Part model, mm, in its own coordinate system. Face numbers are marked on the shaded views. A direction names the side the tool comes from. Coordinates: 2 decimals unless noted, no trailing zeros. Write each loop counter-clockwise with the first axis right and the second up, starting at its lowest first coordinate (ties: lowest second). Pieces come first, ordered by that corner, then holes. Notation, with made-up numbers: (88.5, -33) -> (108.5, -33) arc R17 ccw to (108.5, -27) -> close; hole circle Ø7 at (82.5, 83). An arc over 180 degrees is marked (long way). Write item = value, one per line. Start each with the question number.
Q1. Band-saw the part on A-A, the plane z = 1.75. List the corners of the cut face in (x, y), plus the area to 3 significant figures.
Q2. Band-saw the part on D-D, the plane z = -0.5. Give the number of separate pieces and of enclosed holes in the cut face, plus the area to 3 significant figures.
Q3. Pull direction X, two halves, no side cores. Call the marked faces 1, 2 and 3: released by +X, released by -X, zero draft, split by the parting line, or undercut.
Q4. Band-saw the part on C-C, the plane y = 2.55. List the corners of the cut face in (x, z).
Q5. Band-saw the part on B-B, the plane x = -1.25. List the corners of the cut face in (y, z), plus the area to 3 significant figures.
Q6. Probe line 1 (X direction, y = 0.65, z = 3); line 2 (Z direction, x = 4.25, y = 1.8). List the from-to ranges inside material, lowest first.
Q7. Tool access for the marked faces 4 and 5: list every direction of +Z, -Z, +X, -X, +Y, -Y with a clear straight run to the whole face (end or side of a thin tool).
Autodesk Inventor part; units mm, degrees
ref_plane "YZ Plane" through (0, 0, 0) normal (1, 0, 0) x (0, 1, 0)
ref_plane "XZ Plane" through (0, 0, 0) normal (0, 1, 0) x (-1, 0, 0)
ref_plane "XY Plane" through (0, 0, 0) normal (0, 0, 1) x (1, 0, 0)
sketch "Sketch1" plane through (0, 0, 0) normal (0, 1, 0) x (-1, 0, 0)
  line L0 (5, 5) -> (-5, 5)
  line L1 (-5, 5) -> (-5, -5)
  line L2 (-5, -5) -> (5, -5)
  line L3 (5, -5) -> (5, 5)
  line L4 (6, 6) -> (-6, 6)
  line L5 (-6, 6) -> (-6, -6)
  line L6 (-6, -6) -> (6, -6)
  line L7 (6, -6) -> (6, 6)
  point P0 (0, 0)
  dimension "d0" = 10
  dimension "d1" = 10
  dimension "d2" = 5
  dimension "d3" = 5
  dimension "d4" = 12
  dimension "d5" = 12
  dimension "d6" = 1
  dimension "d7" = 1
extrude "Extrusion1" add sketch "Sketch1" along normal blind 2
sketch "Sketch2" plane through (6, 0, 6) normal (1, 0, 0) x (0, 0, -1)
  line L0 (0, 0) -> (0, 2)
  line L1 (12, 0) -> (12, 2)
  line L2 (0, 2) -> (12, 2)
  line L3 (12, 2) -> (12, 1)
  line L4 (12, 1) -> (0, 1)
  line L5 (0, 1) -> (0, 2)
  point P0 (6, 0)
extrude "Extrusion2" add sketch "Sketch2" against normal blind 11.5
sketch "Sketch3" plane through (0, 2, 0) normal (0, 1, 0) x (1, 0, 0)
  line L0 (-2, -2) -> (2, -2)
  line L1 (2, -2) -> (2, 2)
  line L2 (2, 2) -> (-2, 2)
  line L3 (-2, 2) -> (-2, -2)
  circle A0 centre (0, 0) radius 2.8284
  line L4 (0, -2.8284) -> (-2.8284, 0)
  line L5 (-2.8284, 0) -> (0, 2.8284)
  line L6 (2.8284, 0) -> (0, 2.8284)
  line L7 (2.8284, 0) -> (0, -2.8284)
  point P0 (0.8284, -2)
  point P1 (2, -0.8284)
  point P2 (2, 0.8284)
  point P3 (0.8284, 2)
  point P4 (-0.8284, 2)
  point P5 (-2, 0.8284)
  point P6 (-2, -0.8284)
  point P7 (-0.8284, -2)
  dimension "d13" = 4
  dimension "d14" = 4
  dimension "d15" = 2
  dimension "d16" = 2
extrude "Extrusion3" cut sketch "Sketch3" along normal blind 23.25 and the other way blind 11.625 contours L4 L3 L5 L2 L6 L1 L7 L0
sketch "Sketch4" plane through (0, 2, 0) normal (0, 1, 0) x (1, 0, 0)
  line L0 (2, -0.8284) -> (2, 0.8284)
  line L1 (2, -0.8284) -> (2.8765, -0.8284)
  line L2 (2.8765, -0.8284) -> (2.8765, 0.8284)
  line L3 (2.8765, 0.8284) -> (2, 0.8284)
  line L4 (2, 0.8284) -> (2, -0.8284)
  line L5 (2.8765, -0.8284) -> (7.5124, -0.8284)
  line L6 (7.5124, -0.8284) -> (7.5124, 0.8284)
  line L7 (7.5124, 0.8284) -> (2.8765, 0.8284)
  line L8 (2.8765, 0.8284) -> (2.8765, -0.8284)
  point P0 (0, 0)
  point P1 (2.8765, 0.8284)
  point P2 (2, 0.8284)
extrude "Extrusion4" cut sketch "Sketch4" against normal blind 1
sketch "Sketch5" plane through (0, 2, 0) normal (0, 1, 0) x (1, 0, 0)
  line L0 (-6, -6) -> (6, -6)
  line L1 (6, 0.8284) -> (6, 6)
  line L2 (-6, -6) -> (6, -6)
  line L3 (6, -6) -> (6, 6)
  line L4 (6, 6) -> (-6, 6)
  line L5 (-6, 6) -> (-6, -6)
  point P0 (0, 0)
  point P1 (6, -6)
extrude "Extrusion5" add sketch "Sketch5" along normal blind 25
sketch "Sketch6" plane through (6, 0, 6) normal (1, 0, 0) x (0, 0, -1)
  line L0 (5.1716, 1) -> (5.1716, 2)
  line L1 (5.1716, 2) -> (-3.596, 2)
  line L2 (0, 0) -> (0, 27)
  line L3 (4, 2) -> (5.1716, 2)
  line L4 (5.1716, 2) -> (16.1787, 2)
  line L5 (5.1716, 2) -> (6.8284, 2)
  line L6 (6, 2) -> (6, 6)
  line L7 (0, 2) -> (6, 4)
  line L8 (6, 4) -> (12, 2)
  line L9 (12, 0) -> (12, 27)
  line L10 (12, 2) -> (-2.4689, 2)
  line L11 (-2.4689, 2) -> (-2.4689, 28.669)
  line L12 (-2.4689, 28.669) -> (12, 28.669)
  line L13 (12, 28.669) -> (12, 2)
  point P0 (6, 0)
  dimension "d23" = 4
extrude "Extrusion6" cut sketch "Sketch6" against normal blind 23.25 contours L1 L11 L12 L13 L9 L8 L7
sketch "Sketch7" plane through (-6, 0, 6) normal (0, 0, 1) x (1, 0, 0)
  line L0 (6, 0) -> (6, 4)
  line L1 (12, 4) -> (0, 4)
  line L2 (0, 2) -> (12, 2)
  line L3 (12, 2) -> (6, 4)
  line L4 (0, 4) -> (0, 2)
  line L5 (6, 4) -> (0, 2)
  line L6 (0, 2) -> (13.6732, 2)
  line L7 (13.6732, 2) -> (13.6732, 4.9606)
  line L8 (13.6732, 4.9606) -> (0, 4.9606)
  line L9 (0, 4.9606) -> (0, 2)
extrude "Extrusion7" cut sketch "Sketch7" against normal blind 41.75 contours L5 L4 L1 | L1 L9 L8 L7 L6 L3
sketch "Sketch8" plane through (0, 2, 0) normal (0, -1, 0) x (1, 0, 0)
  line L0 (6, 6) -> (0, 0)
  line L1 (1.9974, 1.9974) -> (-2.0026, 1.9974)
  line L2 (-2.0026, 1.9974) -> (-2.0026, -2.0026)
  line L3 (-2.0026, -2.0026) -> (1.9974, -2.0026)
  line L4 (1.9974, -2.0026) -> (1.9974, 1.9974)
  dimension "d30" = 4
  dimension "d31" = 4
extrude "Extrusion8" cut sketch "Sketch8" against normal blind 105
sketch "Sketch9" plane through (-6, 0, 6) normal (0, 0, 1) x (1, 0, 0)
  line L0 (8, 1) -> (6.8284, 1)
  line L1 (6, 0) -> (7.1, 0)
  line L2 (7.1, 0) -> (7.1, 1)
  line L3 (7.1, 1) -> (6, 1)
  line L4 (6, 1) -> (6, 0)
  line L5 (5.1716, 1) -> (4, 1)
  line L6 (6, 0) -> (4.9, 0)
  line L7 (4.9, 0) -> (4.9, 1)
  line L8 (4.9, 1) -> (6, 1)
  line L9 (6, 1) -> (6, 0)
  dimension "d34" = 1.1
  dimension "d35" = 1.1
extrude "Extrusion9" cut sketch "Sketch9" against normal blind 2.75
equation "\"BendRadius\" = Thickness"
equation "\"BendReliefWidth\" = Thickness"
equation "\"BendReliefDepth\" = 0.5 * Thickness"
equation "\"CornerReliefSize\" = 4 * Thickness"
equation "\"MinimumRemnant\" = 2 * Thickness"
equation "\"TransitionRadius\" = BendRadius"
equation "\"JacobiRadiusSize\" = BendRadius"
equation "\"GapSize\" = Thickness"
properties part number "modelGatePoklice1"
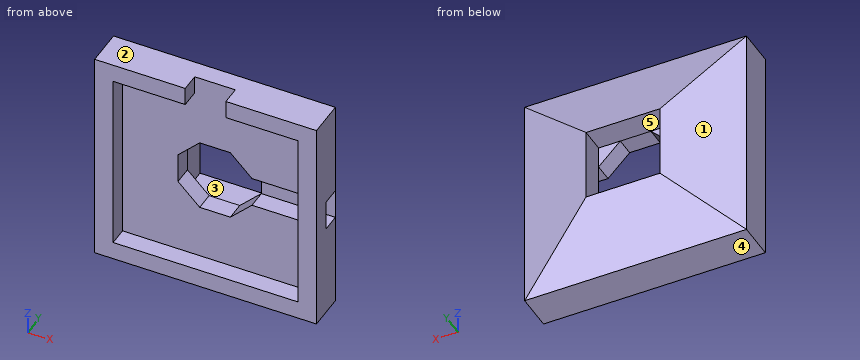
Ans:
q1.outline = (-6, 0) -> (-5, 0) -> (-5, 1) -> (-1.08, 1) -> (-1.08, 2) -> (-2, 2) -> (-2, 3.33) -> (-6, 2) -> close; (1.08, 1) -> (5, 1) -> (5, 0) -> (6, 0) -> (6, 2) -> (2, 3.33) -> (2, 2) -> (1.08, 2) -> close
q1.area = 17.2 mm2
q2.separate_pieces = 3
q2.enclosed_holes = 0
q2.area = 11.3 mm2
q3.face_1 = released by -X
q3.face_2 = zero draft
q3.face_3 = undercut
q4.outline = (-4.35, -4.35) -> (4.35, -4.35) -> (4.35, 4.35) -> (-4.35, 4.35) -> close; hole (-2, -2) -> (2, -2) -> (2, 2) -> (-2, 2) -> close
q5.outline = (0, -6) -> (2, -6) -> (3.33, -2) -> (2, -2) -> (2, -1.58) -> (1, -1.58) -> (1, -5) -> (0, -5) -> close; (0, 5) -> (1, 5) -> (1, 1.58) -> (2, 1.58) -> (2, 2) -> (3.33, 2) -> (2, 6) -> (0, 6) -> close
q5.area = 16.2 mm2
q6.line_1 = -6 to -5, 5 to 6
q6.line_2 = -6 to -0.83, 0.83 to 6
q7.face_4 = -Z, +X, -X, +Y, -Y
q7.face_5 = +Y
